Geometry check sheet. Reference: the model listing, model coordinates, mm. Round coordinates to 2 decimals unless told otherwise and drop trailing zeros. Loops run counter-clockwise (first coordinate to the right, second up) from the corner with the lowest first, then second, coordinate; pieces in that order, holes last. Notation, with made-up numbers: (-4.75, 16) -> (17.25, 16) arc R16 ccw to (17.25, 23) -> close; hole circle Ø2 at (6, 28.25). An arc over 180 degrees is marked (long way). Use one line per item in the form item = value.
from build123d import *

# Parameters (mm, degrees)
SKETCH1_W           = 38
SKETCH1_H           = 20
SKETCH1_R           = 1.5
BOSS_EXTRUDE1_DEPTH = 5
FILLET1_R           = 3
FILLET2_R           = 3
FILLET3_R           = 3
FILLET4_R           = 3


with BuildPart() as part:
    # Sketch1 → Boss-Extrude1 (new body)
    with BuildSketch(Plane.XY):
        with Locations((4.889250814, 9.866449511)):
            Rectangle(SKETCH1_W, SKETCH1_H)
        with Locations((-11.110749186, 15.16286645)):
            Circle(SKETCH1_R, mode=Mode.SUBTRACT)
        with Locations((-11.110749186, 3.651465798)):
            Circle(SKETCH1_R, mode=Mode.SUBTRACT)
        with Locations((20.889250814, 15.16286645)):
            Circle(SKETCH1_R, mode=Mode.SUBTRACT)
        with Locations((20.889250814, 3.651465798)):
            Circle(SKETCH1_R, mode=Mode.SUBTRACT)
    extrude(amount=BOSS_EXTRUDE1_DEPTH)

    # Fillet1
    fillet1_edges = [part.edges().sort_by_distance(p)[0] for p in [
        (23.889250814, 19.866449511, 2.5),
    ]]
    fillet(fillet1_edges, radius=FILLET1_R)

    # Fillet2
    fillet2_edges = [part.edges().sort_by_distance(p)[0] for p in [
        (23.889250814, -0.133550489, 2.5),
    ]]
    fillet(fillet2_edges, radius=FILLET2_R)

    # Fillet3
    fillet3_edges = [part.edges().sort_by_distance(p)[0] for p in [
        (-14.110749186, -0.133550489, 2.5),
    ]]
    fillet(fillet3_edges, radius=FILLET3_R)

    # Fillet4
    fillet4_edges = [part.edges().sort_by_distance(p)[0] for p in [
        (-14.110749186, 19.866449511, 2.5),
    ]]
    fillet(fillet4_edges, radius=FILLET4_R)


solid = part.part
1. Material ranges on line 1 along X through (y, z) = (4, 1.35); line 2 along X through (y, z) = (16.5, 4.55); line 3 along Y through (x, z) = (-10, 2.15), recorded low to high.
Return value:
line_1 = -14.11 to -12.57, -9.65 to 19.43, 22.35 to 23.89
line_2 = -14.11 to -11.79, -10.43 to 20.21, 21.57 to 23.89
line_3 = -0.13 to 2.64, 4.66 to 14.15, 16.17 to 19.87
2. Section check A-A (y = 15.75). Record the boundary of the cut face in (x, z), then the cut area to 3 significant figures.
Return value:
outline = (-14.11, 0) -> (-12.49, 0) -> (-12.49, 5) -> (-14.11, 5) -> close; (-9.73, 0) -> (19.51, 0) -> (19.51, 5) -> (-9.73, 5) -> close; (22.27, 0) -> (23.89, 0) -> (23.89, 5) -> (22.27, 5) -> close
area = 162 mm2
3. Mould release check, pull along Y, two halves, no side actions. Record for faces 1 (the flat face through (5, -0.134, 2)), 2 (the cylindrical face through (-12.216, 16.177, 2.465)), 3 (the flat face through (5, 10, 0)): released by +Y, released by -Y, zero draft, split by the parting line, or undercut.
Return value:
face_1 = released by -Y
face_2 = undercut
face_3 = zero draft
4. Section check B-B (x = -10.5). Record the boundary of the cut face in (y, z), then the cut area to 3 significant figures.
Return value:
outline = (-0.13, 0) -> (2.28, 0) -> (2.28, 5) -> (-0.13, 5) -> close; (5.02, 0) -> (13.79, 0) -> (13.79, 5) -> (5.02, 5) -> close; (16.53, 0) -> (19.87, 0) -> (19.87, 5) -> (16.53, 5) -> close
area = 72.6 mm2
5. Section check C-C (z = 0.5). Record the boundary of the cut face in (x, y).
Return value:
outline = (-14.11, 2.87) arc R3 ccw to (-11.11, -0.13) -> (20.89, -0.13) arc R3 ccw to (23.89, 2.87) -> (23.89, 16.87) arc R3 ccw to (20.89, 19.87) -> (-11.11, 19.87) arc R3 ccw to (-14.11, 16.87) -> close; hole circle Ø3 at (-11.11, 3.65); hole circle Ø3 at (-11.11, 15.16); hole circle Ø3 at (20.89, 3.65); hole circle Ø3 at (20.89, 15.16)
6. Gauge pin test, flat end, axial feed: pin 1 (2.5 mm diameter, centred on x = -11.11, y = 3.65, fed in from +Z). Record the tip position at first contact, or that the pin passes through.
Return value:
pin_1 = through
